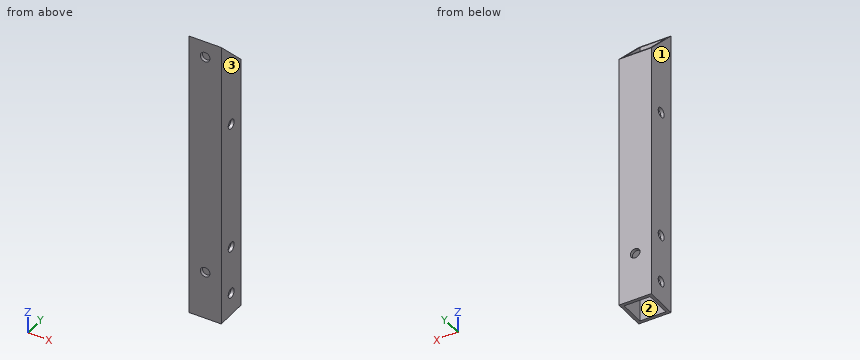
from build123d import *

# Parameters (mm, degrees)
SKETCH_1_W          = 10
SKETCH_1_H          = 10
SKETCH_1_W_2        = 8
SKETCH_1_H_2        = 8
EXTRUDE_1_DEPTH     = 90
SKETCH_2_R          = 1.5
CUT_EXTRUDE_1_DEPTH = 11
SKETCH_3_R          = 1.5
CUT_EXTRUDE_3_DEPTH = 11
CUT_EXTRUDE_4_DEPTH = 10


with BuildPart() as part:
    # 草图1 → 拉伸-薄壁1 (new body)
    with BuildSketch(Plane.XY):
        Rectangle(SKETCH_1_W, SKETCH_1_H)
        Rectangle(SKETCH_1_W_2, SKETCH_1_H_2, mode=Mode.SUBTRACT)
    extrude(amount=EXTRUDE_1_DEPTH)

    # 草图2 → 切除-拉伸1 (cut, through all)
    with BuildSketch(Plane(origin=(5, 0, 0), x_dir=(0, 0, -1), z_dir=(1, 0, 0))):
        with Locations((-62, 0)):
            Circle(SKETCH_2_R)
        with Locations((-7, 0)):
            Circle(SKETCH_2_R)
        with Locations((-22, 0)):
            Circle(SKETCH_2_R)
    extrude(amount=-CUT_EXTRUDE_1_DEPTH, mode=Mode.SUBTRACT)

    # 草图3 → 切除-拉伸3 (cut, through all)
    with BuildSketch(Plane(origin=(0, 5, 0), x_dir=(1, 0, 0), z_dir=(0, 1, 0))):
        with Locations((0, -15)):
            Circle(SKETCH_3_R)
        with Locations((0, -85)):
            Circle(SKETCH_3_R)
    extrude(amount=-CUT_EXTRUDE_3_DEPTH, mode=Mode.SUBTRACT)

    # 草图4 → 切除-拉伸4 (cut)
    with BuildSketch(Plane.ZY.offset(5)):
        Polygon((90, -5), (80, 5), (90, 5), align=None)
    extrude(amount=-CUT_EXTRUDE_4_DEPTH, mode=Mode.SUBTRACT)


solid = part.part
Input: part model. Units: mm. Frame: model coordinates. Face numbers are marked on the shaded views. Round coordinates to 2 decimals unless told otherwise and drop trailing zeros. Loops run counter-clockwise (first coordinate to the right, second up) from the corner with the lowest first, then second, coordinate; pieces in that order, holes last. Notation, with made-up numbers: (72.5, 24.5) -> (108.5, 24.5) arc R22 cw to (108.5, 51.5) -> close; hole circle Ø5 at (85.5, -33.75). An arc over 180 degrees is marked (long way). Answer as a JSON object with one key per item and string values. Group by question number.
1) Ray query, L1, parallel to Y at x = 1, z = 65; L2, parallel to Y at x = 4.6, z = 22. Return the intervals inside material, ascending.
2) Section query D-D on y = -2.75. Output: boundary loops of the cut face in (x, z), plus the area to 4 significant figures.
3) Section query C-C on z = 56. Output: boundary loops of the cut face in (x, y).
4) Draft query along X for the marked faces 1, 2 and 3. Return one class per face: +X half, -X half, draft (parallel to the pull), parting line (faces both ways), or undercut.
5) Pin query (flat end, axial travel): pin 1 (4 mm diameter, centred on x = 0, z = 15, fed in from -Y); pin 2 (3 mm diameter, centred on x = -4, y = 3.5, fed in from +Z). Return the tip coordinate at first contact, or that it passes through.
6) Section query A-A on y = 2.25. Output: boundary loops of the cut face in (x, z), plus the area to 4 significant figures.
7) Section query B-B on z = 85. Output: boundary loops of the cut face in (x, y).
Reply:
{
 "1": {"L1": "y = -5 to -4, 4 to 5", "L2": "y = -5 to -1.5, 1.5 to 5"},
 "2": {"outline": "(-5, 0) -> (-4, 0) -> (-4, 87.75) -> (-5, 87.75) -> close; (4, 0) -> (5, 0) -> (5, 87.75) -> (4, 87.75) -> close", "area": "175.5 mm2"},
 "3": {"outline": "(-5, -5) -> (5, -5) -> (5, 5) -> (-5, 5) -> close; hole (-4, -4) -> (4, -4) -> (4, 4) -> (-4, 4) -> close"},
 "4": {"face 1": "-X half", "face 2": "undercut", "face 3": "+X half"},
 "5": {"pin 1": "stops at y = -5", "pin 2": "stops at z = 83"},
 "6": {"outline": "(-5, 0) -> (-4, 0) -> (-4, 82.75) -> (-5, 82.75) -> close; (4, 0) -> (5, 0) -> (5, 82.75) -> (4, 82.75) -> close", "area": "165.5 mm2"},
 "7": {"outline": "(-5, -5) -> (-1.5, -5) -> (-1.5, -4) -> (-4, -4) -> (-4, 0) -> (-5, 0) -> close; (1.5, -5) -> (5, -5) -> (5, 0) -> (4, 0) -> (4, -4) -> (1.5, -4) -> close"}
}
